Geometry check sheet. Reference: the model listing, model coordinates, mm. Face numbers are marked on the shaded views. A direction names the side the tool comes from. Round coordinates to 2 decimals unless told otherwise and drop trailing zeros. Order: outer loops, then holes, each group sorted by start corner. A loop starts at its lowest first (then second) coordinate and runs counter-clockwise, first axis right, second up.
(1) Release check for a two-part mould opening along X. For the marked faces 1, 2 and 3 record: +X half, -X half, draft (parallel to the pull), parting line (faces both ways), or undercut.
(2) Sectioned sample at C-C (z = 4.75). Record the boundary of the cut face in (x, y), plus the area to 3 significant figures.
(3) Sectioned sample at B-B (y = 0). Record the boundary of the cut face in (x, z), plus the area to 3 significant figures.
(4) Go/stop test with flat-tipped pins: pin 1 (3 mm diameter, centred on y = -4, z = 2, fed in from -X); pin 2 (1 mm diameter, centred on y = -1, z = 3, fed in from +X). Record where each tip stops, or that it passes through.
(5) Sectioned sample at D-D (y = 6). Record the boundary of the cut face in (x, z), plus the area to 3 significant figures.
(6) Set-up check for the marked faces 4, 5 and 6: record each of +Z, -Z, +X, -X, +Y, -Y from which the full face is reachable in a straight line by a thin tool's end or side.
(7) Material ranges on line 1 along Y through (x, z) = (0, 9.75); line 2 along Y through (x, z) = (-0.25, 4); line 3 along X through (y, z) = (6, 9), recorded low to high.
(8) Sectioned sample at A-A (x = 0). Record the boundary of the cut face in (y, z).
from build123d import *

# Parameters (mm, degrees)
SCHIZZO1_R                   = 7.5
SCHIZZO1_R_2                 = 2.5
ESTRUSIONE_ESTRUSIONE1_DEPTH = 15
ESTRUSIONE_ESTRUSIONE2_DEPTH = 6
ESTRUSIONE_ESTRUSIONE3_START = -9
SCHIZZO3_R                   = 2.5
SCHIZZO3_R_2                 = 2.35
ESTRUSIONE_ESTRUSIONE3_DEPTH = 9


with BuildPart() as part:
    # Schizzo1 → Estrusione-Estrusione1 (new body)
    with BuildSketch(Plane.XY):
        Circle(SCHIZZO1_R)
        Circle(SCHIZZO1_R_2, mode=Mode.SUBTRACT)
    extrude(amount=ESTRUSIONE_ESTRUSIONE1_DEPTH)

    # Schizzo2 → Estrusione-Estrusione2 (add)
    with BuildSketch(Plane(origin=(0, 0, 0), x_dir=(-1, 0, 0), z_dir=(0, 0, -1))):
        with BuildLine():
            Line((-2, -1.5), (2, -1.5))
            ThreePointArc((2, -1.5), (0, -2.5), (-2, -1.5))
        make_face()
        with BuildLine():
            Line((-2, 1.5), (2, 1.5))
            ThreePointArc((2, 1.5), (0, 2.5), (-2, 1.5))
        make_face()
    extrude(amount=-ESTRUSIONE_ESTRUSIONE2_DEPTH)

    # Schizzo3 → Estrusione-Estrusione3 (add)
    with BuildSketch(Plane.XY.offset(15).offset(ESTRUSIONE_ESTRUSIONE3_START)):
        Circle(SCHIZZO3_R)
        Circle(SCHIZZO3_R_2, mode=Mode.SUBTRACT)
    extrude(amount=ESTRUSIONE_ESTRUSIONE3_DEPTH)


solid = part.part
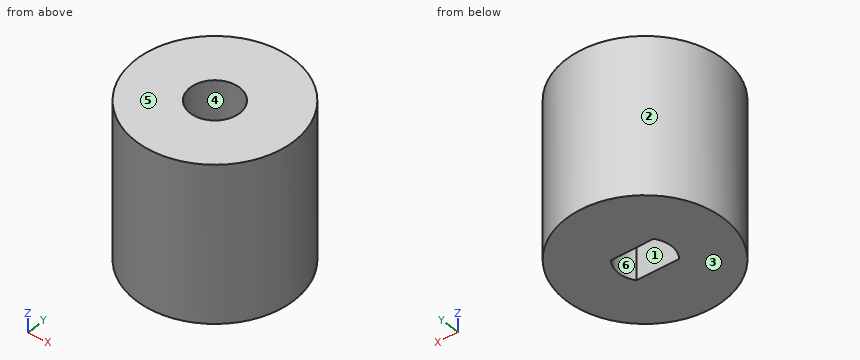
Answer below:
1. face 1: undercut
1. face 2: parting line
1. face 3: draft
2. outline: circle Ø15 at (0, 0); hole (-2, -1.5) - (2, -1.5) arc R2.5 ccw to (2, 1.5) - (-2, 1.5) arc R2.5 ccw to start
2. area: 163 mm2
3. outline: (-7.5, 0) - (-2.5, 0) - (-2.5, 6) - (-2.35, 6) - (-2.35, 15) - (-7.5, 15) - close; (2.35, 6) - (2.5, 6) - (2.5, 0) - (7.5, 0) - (7.5, 15) - (2.35, 15) - close
3. area: 153 mm2
4. pin 1: stops at x = -7.07
4. pin 2: stops at x = 7.48
5. outline: (-4.5, 0) - (4.5, 0) - (4.5, 15) - (-4.5, 15) - close
5. area: 135 mm2
6. face 4: +Z
6. face 5: +Z, +X, -X, +Y, -Y
6. face 6: -Z
7. line 1: y = -7.5 to -2.35, 2.35 to 7.5
7. line 2: y = -7.5 to -1.5, 1.5 to 7.5
7. line 3: x = -4.5 to 4.5
8. outline: (-7.5, 0) - (-1.5, 0) - (-1.5, 6) - (-2.35, 6) - (-2.35, 15) - (-7.5, 15) - close; (1.5, 0) - (7.5, 0) - (7.5, 15) - (2.35, 15) - (2.35, 6) - (1.5, 6) - close
